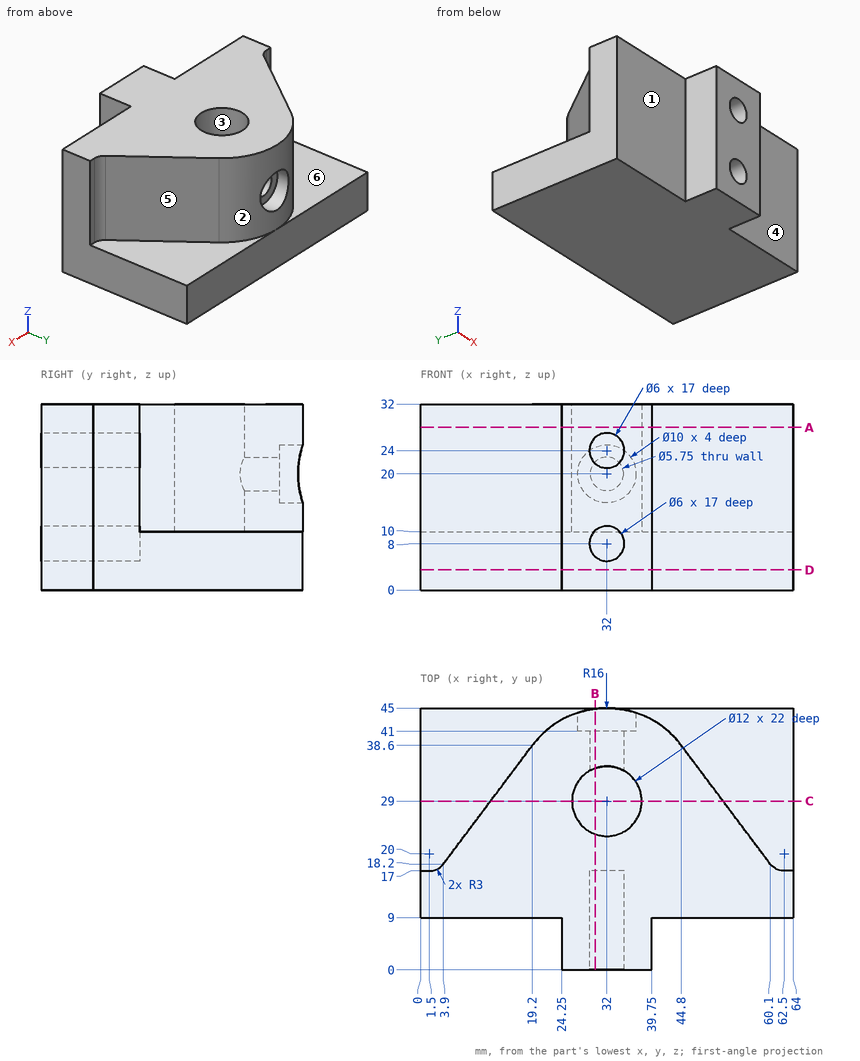
Could you check a few things on this drawing? It's one solid part, dimensions in mm from its lowest x, y, z. A direction names the side the tool comes from. Round coordinates to 2 decimals unless told otherwise and drop trailing zeros. Loops run counter-clockwise (first coordinate to the right, second up) from the corner with the lowest first, then second, coordinate; pieces in that order, holes last. Notation, with made-up numbers: M 86,49 L 103,49 A19 cw 103,55 Z; hole C 28.25,52 d4. An arc over 180 degrees is marked long. Write each question's results on one line, items separated by ' | '. Start each with the question number.
(1) I want a section at B-B (x = 30). Please give me the cut outline in (y, z).
(2) I want a section at D-D (z = 3.5). Please give me the cut outline in (x, y).
(3) On a 3-axis mill with a long thin cutter (end or side, diameter ignored), from which of +Z, -Z, +X, -X, +Y, -Y can I reach the whole of each face in a straight line? I mean the marked faces 4, 5 and 6. Say none if no direction works.
(4) If I drill on probe 1 along Z at (x, y) = (32, 12); probe 2 along Z at (x, y) = (32, 43.4); probe 3 along Y at (x, z) = (10.5, 29), over which ranges is the centre line in solid material (lowest first)? Write a range as from..to.
(5) I want a section at A-A (z = 28). Please give me the cut outline in (x, y).
(6) I want a section at C-C (y = 29). Please give me the cut outline in (x, z), then the cut area to 3 significant figures.
(7) Thinking about a two-plate mould opening in Y: for the marked faces 1, 2 and 3, which applies, pulls with the +Y half, pulls with the -Y half, needs draft (parallel to the pull), parting line crosses it, or undercut?
(8) Will these pins go through, and if not, where does the flat tip stop? P1, Ø4.5, axis at y = 6, z = 15, coming from the +X side; P2, Ø1.5, axis at x = 41, z = 14.5, coming from the +Y side; P3, Ø3.5, axis at x = 32, z = 20, coming from the +Y side.
Solved:
1) outline: M 0,0 L 45,0 L 45,10 L 44.87,10 L 44.87,15.42 L 41,15.42 L 41,17.93 L 34.66,17.93 L 34.66,10 L 23.34,10 L 23.34,32 L 0,32 L 0,26.24 L 17,26.24 L 17,21.76 L 0,21.76 L 0,10.24 L 17,10.24 L 17,5.76 L 0,5.76 Z; M 34.66,22.07 L 41,22.07 L 41,24.58 L 44.87,24.58 L 44.87,32 L 34.66,32 Z
2) outline: M 0,9 L 24.25,9 L 24.25,0 L 39.75,0 L 39.75,9 L 64,9 L 64,45 L 0,45 Z
3) face 4: +Z, -Z, +X, -Y | face 5: +Z, +X, +Y | face 6: +Z, -X, +Y
4) probe 1: z = 0..5, 11..21, 27..32 | probe 2: z = 0..15, 25..32 | probe 3: y = 9..27
5) outline: M 0,9 L 24.25,9 L 24.25,0 L 39.75,0 L 39.75,9 L 64,9 L 64,17 L 62.5,17 A3 cw 60.1,18.2 L 44.8,38.6 A16 ccw 19.2,38.6 L 3.9,18.2 A3 cw 1.5,17 L 0,17 Z; hole C 32,29 d12
6) outline: M 0,0 L 64,0 L 64,10 L 52,10 L 52,32 L 38,32 L 38,10 L 26,10 L 26,32 L 12,32 L 12,10 L 0,10 Z | area: 1,260 mm²
7) face 1: pulls with the -Y half | face 2: pulls with the +Y half | face 3: undercut
8) P1: stops at x = 39.75 | P2: stops at y = 42.71 | P3: stops at y = 23.26
